CAD build for the part. Positions are in the model's coordinates, mm. Face numbers are marked on the shaded views. A direction names the side the tool comes from. Give positions to 0.01 mm unless a question says otherwise; leave off trailing zeros. Loops run counter-clockwise (first coordinate to the right, second up) from the corner with the lowest first, then second, coordinate; pieces in that order, holes last. Notation, with made-up numbers: (68.5, 13) - (103.5, 13) arc R13 cw to (103.5, 18) - close; hole circle Ø9 at (24, 38.5). An arc over 180 degrees is marked (long way). Return JSON: item names as keys, results as strings.
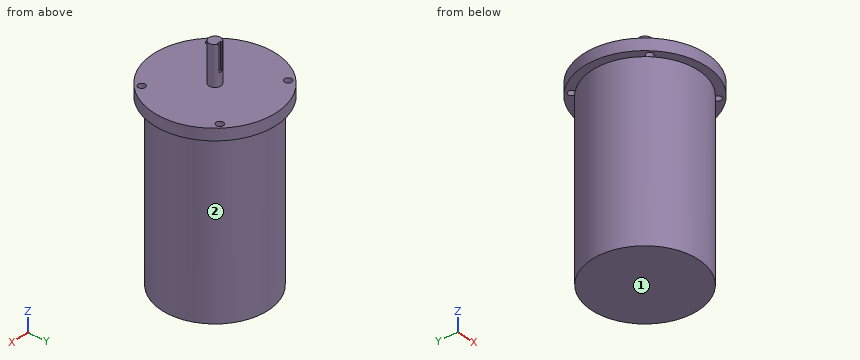
from build123d import *

# Parameters (mm, degrees)
SKETCH2_R           = 71.501
BOSS_EXTRUDE1_DEPTH = 231.199972222
SKETCH3_R           = 82.55
SKETCH3_R_2         = 4.7625
BOSS_EXTRUDE2_DEPTH = 15.434027778
SKETCH4_R           = 7.9375
BOSS_EXTRUDE3_DEPTH = 52.324
SKETCH5_W           = 4.826
SKETCH5_H           = 4.826
CUT_EXTRUDE1_DEPTH  = 35.052


with BuildPart() as part:
    # Sketch2 → Boss-Extrude1 (new body)
    with BuildSketch(Plane.XY):
        Circle(SKETCH2_R)
    extrude(amount=BOSS_EXTRUDE1_DEPTH)

    # Sketch3 → Boss-Extrude2 (add)
    with BuildSketch(Plane.XY.offset(231.199972222)):
        Circle(SKETCH3_R)
        with Locations((-52.714065184, 52.803905992)):
            Circle(SKETCH3_R_2, mode=Mode.SUBTRACT)
        with Locations((52.803905992, 52.714065184)):
            Circle(SKETCH3_R_2, mode=Mode.SUBTRACT)
        with Locations((52.714065184, -52.803905992)):
            Circle(SKETCH3_R_2, mode=Mode.SUBTRACT)
        with Locations((-52.803905992, -52.714065184)):
            Circle(SKETCH3_R_2, mode=Mode.SUBTRACT)
    extrude(amount=BOSS_EXTRUDE2_DEPTH)

    # Sketch4 → Boss-Extrude3 (add)
    with BuildSketch(Plane.XY.offset(246.634)):
        Circle(SKETCH4_R)
    extrude(amount=BOSS_EXTRUDE3_DEPTH)

    # Sketch5 → Cut-Extrude1 (cut)
    with BuildSketch(Plane.XY.offset(298.958)):
        with Locations((0, 7.9375)):
            Rectangle(SKETCH5_W, SKETCH5_H)
    extrude(amount=-CUT_EXTRUDE1_DEPTH, mode=Mode.SUBTRACT)


solid = part.part
1. Which spindle directions (+Z, -Z, +X, -X, +Y, -Y) get a long thin tool onto all of the face, cutting with end or side? Do the marked faces 1 and 2. Say none if no direction does.
Values follow:
{"face 1": "-Z, +X, -X, +Y, -Y", "face 2": "-Z"}
2. Cut at D-D, the plane y = 0. Write the cut outline in (x, z).
Values follow:
{"outline": "(-82.55, 231.2) - (-71.5, 231.2) - (-71.5, 0) - (71.5, 0) - (71.5, 231.2) - (82.55, 231.2) - (82.55, 246.63) - (7.94, 246.63) - (7.94, 298.96) - (-7.94, 298.96) - (-7.94, 246.63) - (-82.55, 246.63) - close"}
3. Cut at A-A, the plane y = -43. Write the cut outline in (x, z).
Values follow:
{"outline": "(-70.47, 231.2) - (-57.13, 231.2) - (-57.13, 0) - (57.13, 0) - (57.13, 231.2) - (70.47, 231.2) - (70.47, 246.63) - (-70.47, 246.63) - close"}
4. Drop flat-ended pins along their axis: P1, Ø1.5, axis at y = -34.5, z = 116, coming from the +X side; P2, Ø4, axis at x = -61.5, z = 231, coming from the +Y side; P3, Ø1, axis at y = 6.5, z = 289, coming from the +X side; P4, Ø5.5, axis at x = -52.8, y = -52.71, coming from the -Z side. Give the stop position or say it passes through.
Values follow:
{"P1": "stops at x = 63.03", "P2": "stops at y = 57.21", "P3": "stops at x = 5.2", "P4": "passes through"}
5. Cut at C-C, the plane x = -37.5. Write the cut outline in (y, z).
Values follow:
{"outline": "(-73.54, 231.2) - (-60.88, 231.2) - (-60.88, 0) - (60.88, 0) - (60.88, 231.2) - (73.54, 231.2) - (73.54, 246.63) - (-73.54, 246.63) - close"}
6. Cut at B-B, the plane z = 98.5. Write the cut outline in (x, y).
Values follow:
{"outline": "circle Ø143 at (0, 0)"}
7. Drill centre lines: probe 1 along Z at (x, y) = (25, -26); probe 2 along X at (y, z) = (0.5, 19.5); probe 3 along X at (y, z) = (0.5, 283). Where is each one in solid material? Low to high.
Values follow:
{"probe 1": "z = 0 to 246.63", "probe 2": "x = -71.5 to 71.5", "probe 3": "x = -7.92 to 7.92"}
